from build123d import *

# Parameters (mm, degrees)
F1_DEPTH = 2
F2_R     = 6
F3_R     = 15


with BuildPart() as f1:
    # F0 (on Top) → F1 (new body)
    with BuildSketch(Plane.XY):
        with BuildLine():
            Line((15, 27.6992779689), (15, 34.8053157432))
            ThreePointArc((15, 34.8053157432), (0, 37.9000000526), (-15, 34.8053157432))
            Line((-15, 34.8053157432), (-15, 27.6992779689))
            ThreePointArc((-15, 27.6992779689), (-13.8963378037, 28.2690961236), (-12.771069404, 28.7949611265))
            ThreePointArc((-12.771069404, 28.7949611265), (-11.9279702901, 30.7688726599), (-9.9746921233, 29.8790146599))
            ThreePointArc((-9.9746921233, 29.8790146599), (0, 31.5), (9.9746921233, 29.8790146599))
            ThreePointArc((9.9746921233, 29.8790146599), (11.6440081906, 30.8478948191), (12.8857898224, 29.370287539))
            ThreePointArc((12.8857898224, 29.370287539), (12.8568301638, 29.0769612466), (12.771069404, 28.7949611265))
            ThreePointArc((12.771069404, 28.7949611265), (13.8963378037, 28.2690961236), (15, 27.6992779689))
        make_face()
        with BuildLine():
            ThreePointArc((-12.771069404, 28.7949611265), (-13.8963378037, 28.2690961236), (-15, 27.6992779689))
            Line((-15, 27.6992779689), (-15, 25.9807621135))
            ThreePointArc((-15, 25.9807621135), (-12.9600924591, 27.0561638717), (-10.8436093232, 27.9717024302))
            ThreePointArc((-10.8436093232, 27.9717024302), (-11.9749780232, 27.9908466145), (-12.771069404, 28.7949611265))
        make_face()
        with BuildLine():
            Line((15, 25.9807621135), (15, 27.6992779689))
            ThreePointArc((15, 27.6992779689), (13.8963378037, 28.2690961236), (12.771069404, 28.7949611265))
            ThreePointArc((12.771069404, 28.7949611265), (11.9749780416, 27.9908466224), (10.8436093607, 27.9717024157))
            ThreePointArc((10.8436093607, 27.9717024157), (12.9600924772, 27.056163863), (15, 25.9807621135))
        make_face()
        with BuildLine():
            Line((-15, -27.6992779689), (-15, -34.8053157432))
            ThreePointArc((-15, -34.8053157432), (0, -37.9000000526), (15, -34.8053157432))
            Line((15, -34.8053157432), (15, -27.6992779689))
            ThreePointArc((15, -27.6992779689), (13.8963378037, -28.2690961236), (12.771069404, -28.7949611265))
            ThreePointArc((12.771069404, -28.7949611265), (12.8568301638, -29.0769612466), (12.8857898224, -29.370287539))
            ThreePointArc((12.8857898224, -29.370287539), (11.6440081906, -30.8478948191), (9.9746921233, -29.8790146599))
            ThreePointArc((9.9746921233, -29.8790146599), (0, -31.5), (-9.9746921233, -29.8790146599))
            ThreePointArc((-9.9746921233, -29.8790146599), (-11.9279702901, -30.7688726599), (-12.771069404, -28.7949611265))
            ThreePointArc((-12.771069404, -28.7949611265), (-13.8963378037, -28.2690961236), (-15, -27.6992779689))
        make_face()
        with BuildLine():
            Line((-15, -25.9807621135), (-15, -27.6992779689))
            ThreePointArc((-15, -27.6992779689), (-13.8963378037, -28.2690961236), (-12.771069404, -28.7949611265))
            ThreePointArc((-12.771069404, -28.7949611265), (-11.9749780659, -27.9908466327), (-10.8436094098, -27.9717023967))
            ThreePointArc((-10.8436094098, -27.9717023967), (-12.960092501, -27.0561638516), (-15, -25.9807621135))
        make_face()
        with BuildLine():
            ThreePointArc((12.771069404, -28.7949611265), (13.8963378037, -28.2690961236), (15, -27.6992779689))
            Line((15, -27.6992779689), (15, -25.9807621135))
            ThreePointArc((15, -25.9807621135), (12.9600924534, -27.0561638744), (10.8436093114, -27.9717024348))
            ThreePointArc((10.8436093114, -27.9717024348), (11.9749780173, -27.990846612), (12.771069404, -28.7949611265))
        make_face()
        with BuildLine():
            ThreePointArc((27, 13.0766968306), (21.968812558, 20.4296665365), (15, 25.9807621135))
            ThreePointArc((15, 25.9807621135), (12.9600924772, 27.056163863), (10.8436093607, 27.9717024157))
            ThreePointArc((10.8436093607, 27.9717024157), (2.01e-08, 30), (-10.8436093232, 27.9717024302))
            ThreePointArc((-10.8436093232, 27.9717024302), (-12.9600924591, 27.0561638717), (-15, 25.9807621135))
            ThreePointArc((-15, 25.9807621135), (-21.968812558, 20.4296665365), (-27, 13.0766968306))
            Line((-27, 13.0766968306), (-27, -13.0766968306))
            ThreePointArc((-27, -13.0766968306), (-21.968812558, -20.4296665365), (-15, -25.9807621135))
            ThreePointArc((-15, -25.9807621135), (-12.960092501, -27.0561638516), (-10.8436094098, -27.9717023967))
            ThreePointArc((-10.8436094098, -27.9717023967), (-5.28e-08, -30), (10.8436093114, -27.9717024348))
            ThreePointArc((10.8436093114, -27.9717024348), (12.9600924534, -27.0561638744), (15, -25.9807621135))
            ThreePointArc((15, -25.9807621135), (21.968812558, -20.4296665365), (27, -13.0766968306))
            Line((27, -13.0766968306), (27, 13.0766968306))
        make_face()
    extrude(amount=F1_DEPTH)

    # F2
    f2_edges = [f1.edges().sort_by_distance(p)[0] for p in [
        (-15, -34.805316, 1),
        (15, -34.805316, 1),
        (15, 34.805316, 1),
        (-15, 34.805316, 1),
        (27, 13.076697, 1),
        (27, -13.076697, 1),
        (-27, 13.076697, 1),
        (-27, -13.076697, 1),
    ]]
    fillet(f2_edges, radius=F2_R)

    # F3
    f3_edges = [f1.edges().sort_by_distance(p)[0] for p in [
        (-15, -25.980762, 1),
        (15, -25.980762, 1),
        (15, 25.980762, 1),
        (-15, 25.980762, 1),
    ]]
    fillet(f3_edges, radius=F3_R)


solid = f1.part
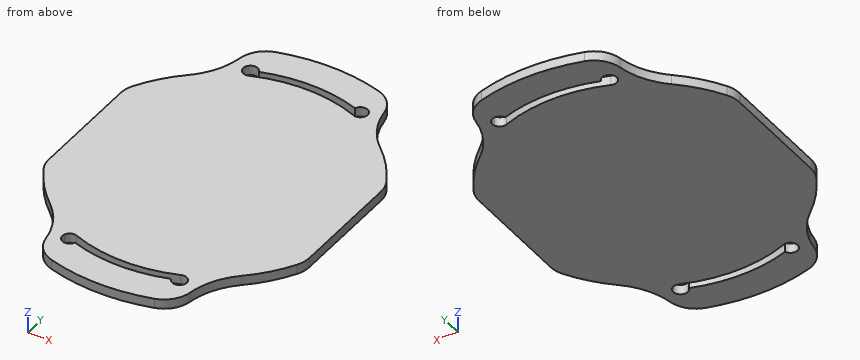
For this review, take the finished solid that the model builds, in its own axes (mm). Round coordinates to 2 decimals unless told otherwise and drop trailing zeros. Loops run counter-clockwise (first coordinate to the right, second up) from the corner with the lowest first, then second, coordinate; pieces in that order, holes last. Notation, with made-up numbers: (82.25, 22.5) - (115.25, 22.5) arc R19 cw to (115.25, 49.5) - close; hole circle Ø7 at (-3, 80.5). An arc over 180 degrees is marked (long way). Put each result on its own line as item: value. Start each with the question number.
1. Consider section C-C on x = 8. State the section outline as (y, z) points.
2. Consider section A-A on x = -1. State the section outline as (y, z) points, plus the area to 3 significant figures.
3. Consider section B-B on z = 1.5. State how many separate pieces and enclosed holes the cut face has, plus the area to 3 significant figures.
4. Consider section D-D on y = -33. State the section outline as (x, z) points.
5. Insertion check: P1, Ø1, axis at x = 10, z = 1.5, coming from the -Y side. The pin has a flat end and moves straight along its axis. Give the tip position at first contact, or say it passes through.
6. For probe 1 along Y at (x, z) = (-2, 1.15); probe 2 along Y at (x, z) = (12.5, 0.15); probe 3 along Y at (x, z) = (-14, 1.55), list the stretches that pass through material, from the lowest coordinate up. Write a range as [from, to].
Result sheet:
1. outline: (-37.05, 0) - (-30.47, 0) - (-30.47, 2) - (-37.05, 2) - close; (-28.91, 0) - (28.91, 0) - (28.91, 2) - (-28.91, 2) - close; (30.47, 0) - (37.05, 0) - (37.05, 2) - (30.47, 2) - close
2. outline: (-37.89, 0) - (-31.48, 0) - (-31.48, 2) - (-37.89, 2) - close; (-29.98, 0) - (29.98, 0) - (29.98, 2) - (-29.98, 2) - close; (31.48, 0) - (37.89, 0) - (37.89, 2) - (31.48, 2) - close
2. area: 146 mm^2
3. separate pieces: 1
3. enclosed holes: 2
3. area: 3,130 mm^2
4. outline: (-14.5, 0) - (14.5, 0) - (14.5, 2) - (-14.5, 2) - close
5. P1: y = -36.69
6. probe 1: [-37.85, -31.44], [-29.93, 29.93], [31.44, 37.85]
6. probe 2: [-35.48, -30.37], [-28.37, 28.37], [30.37, 35.48]
6. probe 3: [-33.92, 33.92]
